Input: dimensioned drawing with shaded views. Units: mm. Origin: part minimum x, y, z. A direction names the side the tool comes from. Give positions to 0.01 mm unless a question says otherwise; leave off trailing zeros. Write each loop counter-clockwise with the first axis right and the second up, starting at its lowest first coordinate (ties: lowest second). Pieces come first, ordered by that corner, then holes.
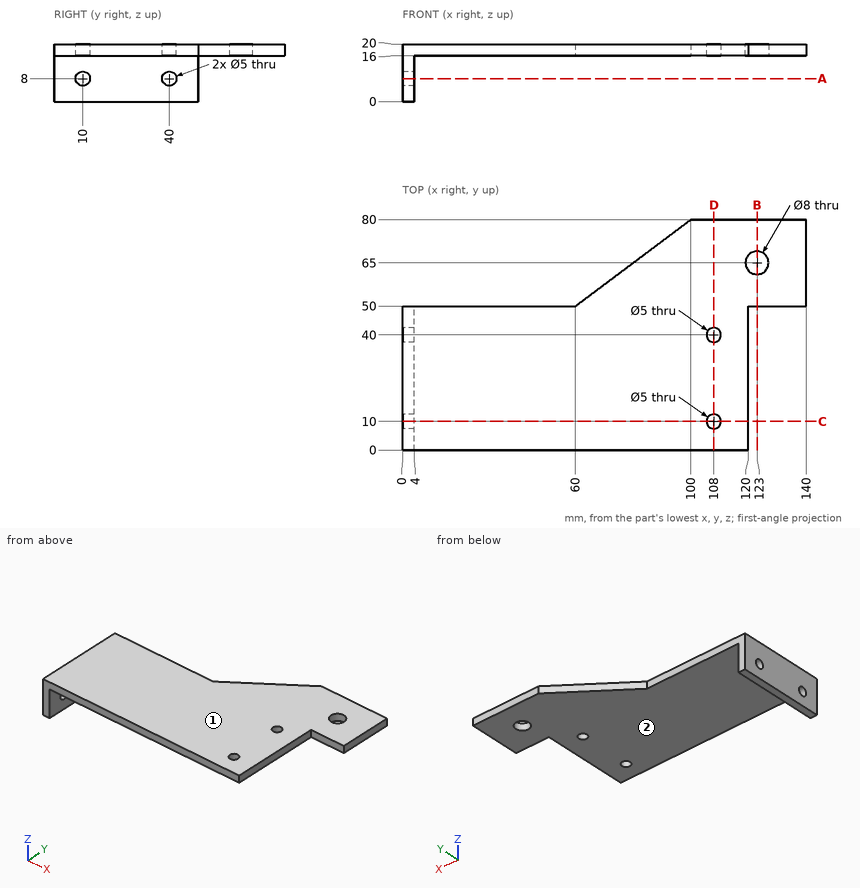
Item 1: Section D-D (x = 108). Return loops of the section in (y, z).
Item 2: Section C-C (y = 10). Return loops of the section in (x, z).
Item 3: Set-up query: the marked faces 1 and 2. Return all of +Z, -Z, +X, -X, +Y, -Y with unobstructed straight access to the full face (end or side cutting, diameter ignored); none if empty.
Item 4: Section A-A (z = 8). Return loops of the section in (x, y), and give its area (3 significant figures).
Item 5: Section B-B (x = 123). Return loops of the section in (y, z), and give its area (3 significant figures).
Item 6: Ray query, line 1 (Y direction, x = 108, z = 18); line 2 (Y direction, x = 1.95, z = 8); line 3 (Y direction, x = 123, z = 17.5). Return the intervals inside material, ascending.
Item 7: Pin query (flat end, axial travel): pin 1 (1 mm diameter, centred on y = 23.5, z = 3, fed in from +X); pin 2 (1.2 mm diameter, centred on x = 132.5, z = 17.5, fed in from -Y); pin 3 (1.5 mm diameter, centred on x = 24.5, y = 27, fed in from -Z); pin 4 (6 mm diameter, centred on y = 10, z = 8, fed in from -X). Return the tip coordinate at first contact, or that it passes through.
Solved:
1. outline: (0, 16) - (7.5, 16) - (7.5, 20) - (0, 20) - close; (12.5, 16) - (37.5, 16) - (37.5, 20) - (12.5, 20) - close; (42.5, 16) - (80, 16) - (80, 20) - (42.5, 20) - close
2. outline: (0, 0) - (4, 0) - (4, 5.5) - (0, 5.5) - close; (0, 10.5) - (4, 10.5) - (4, 16) - (105.5, 16) - (105.5, 20) - (0, 20) - close; (110.5, 16) - (120, 16) - (120, 20) - (110.5, 20) - close
3. face 1: +Z, +X, -X, +Y, -Y
3. face 2: -Z, +X, +Y, -Y
4. outline: (0, 0) - (4, 0) - (4, 7.5) - (0, 7.5) - close; (0, 12.5) - (4, 12.5) - (4, 37.5) - (0, 37.5) - close; (0, 42.5) - (4, 42.5) - (4, 50) - (0, 50) - close
4. area: 160 mm2
5. outline: (50, 16) - (61, 16) - (61, 20) - (50, 20) - close; (69, 16) - (80, 16) - (80, 20) - (69, 20) - close
5. area: 88.0 mm2
6. line 1: y = 0 to 7.5, 12.5 to 37.5, 42.5 to 80
6. line 2: y = 0 to 7.5, 12.5 to 37.5, 42.5 to 50
6. line 3: y = 50 to 61, 69 to 80
7. pin 1: stops at x = 4
7. pin 2: stops at y = 50
7. pin 3: stops at z = 16
7. pin 4: stops at x = 0
